Verification items for the finished model (mm, model axes). Face numbers are marked on the shaded views. A direction names the side the tool comes from. Round coordinates to 2 decimals unless told otherwise and drop trailing zeros. Write each loop counter-clockwise with the first axis right and the second up, starting at its lowest first coordinate (ties: lowest second). Pieces come first, ordered by that corner, then holes.
from build123d import *

# Parameters (mm, degrees)
F0_R     = 12.7
F1_DEPTH = 2.032


with BuildPart() as f1:
    # F0 (on Top) → F1 (new body)
    with BuildSketch(Plane.XY):
        Circle(F0_R)
        with BuildLine():
            ThreePointArc((3.175, 0.155574), (4.57905, -1.610295), (5.08, -3.81))
            ThreePointArc((5.08, -3.81), (-2.199705, -8.38905), (-3.175, 0.155574))
            Line((-3.175, 0.155574), (-3.175, 5.08))
            ThreePointArc((-3.175, 5.08), (0, 8.255), (3.175, 5.08))
            Line((3.175, 5.08), (3.175, 0.155574))
        make_face(mode=Mode.SUBTRACT)
    extrude(amount=F1_DEPTH)


solid = f1.part
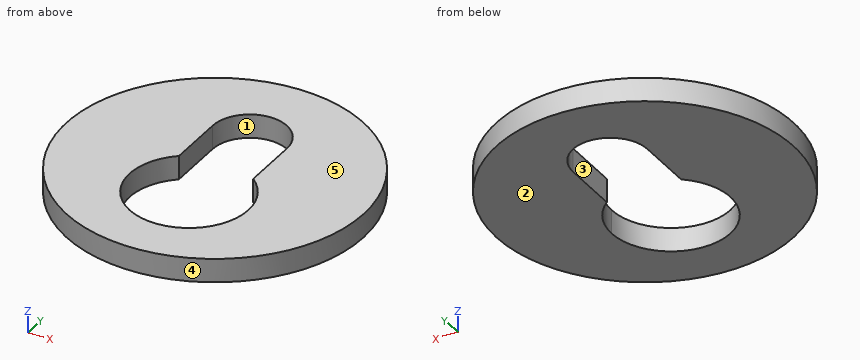
Q1. Release check for a two-part mould opening along Y. For the marked faces 3, 4 and 5 record: released by +Y, released by -Y, zero draft, split by the parting line, or undercut.
Recorded:
face 3: undercut
face 4: split by the parting line
face 5: zero draft
Q2. Sectioned sample at A-A (x = 0). Enter the section's corners in (y, z) (3 decimals).
Recorded:
outline: (-12.7, 0) - (-8.89, 0) - (-8.89, 2.032) - (-12.7, 2.032) - close; (8.255, 0) - (12.7, 0) - (12.7, 2.032) - (8.255, 2.032) - close
Q3. Sectioned sample at B-B (z = 0.5). Enter the section's corners in (x, y) (3 decimals), plus the area to 3 significant figures.
Recorded:
outline: circle Ø25.4 at (0, 0); hole (-3.175, 0.156) arc R5.08 ccw (long way) to (3.175, 0.156) - (3.175, 5.08) arc R3.175 ccw to (-3.175, 5.08) - close
area: 383 mm2
Q4. Sectioned sample at C-C (y = -2.25). Enter the section's corners in (x, z).
Recorded:
outline: (-12.5, 0) - (-4.83, 0) - (-4.83, 2.03) - (-12.5, 2.03) - close; (4.83, 0) - (12.5, 0) - (12.5, 2.03) - (4.83, 2.03) - close
Q5. Sectioned sample at D-D (y = -11). Enter the section's corners in (x, z), plus the area to 3 significant figures.
Recorded:
outline: (-6.35, 0) - (6.35, 0) - (6.35, 2.03) - (-6.35, 2.03) - close
area: 25.8 mm2
Q6. Tool access check on the marked faces 1 and 2. Record the directions out of +Z, -Z, +X, -X, +Y, -Y that give a thin tool (end or side, any length) a straight path to the whole face; none if there is none.
Recorded:
face 1: +Z, -Z
face 2: -Z, +X, -X, +Y, -Y
Q7. Depth check by flat-ended pin: P1, Ø1, axis at x = 7.5, z = 0.5, coming from the +Y side; P2, Ø2, axis at x = -7.5, y = -6, coming from the -Z side; P3, Ø1, axis at y = 3, z = 0.5, coming from the +X side; P4, Ø1, axis at y = 2, z = 1.5, coming from the -X side. Enter the tip coordinate at first touch or a pass-through.
Recorded:
P1: stops at y = 10.6
P2: stops at z = 0
P3: stops at x = 12.45
P4: stops at x = -12.61
Q8. Material ranges on line 1 along Y through (x, z) = (0, 1.15) (3 decimals); line 2 along X through (y, z) = (-3, 1.75) (3 decimals); line 3 along Y through (x, z) = (-2.5, 1.9), recorded low to high.
Recorded:
line 1: y = -12.7 to -8.89, 8.255 to 12.7
line 2: x = -12.341 to -5.015, 5.015 to 12.341
line 3: y = -12.45 to -8.23, 7.04 to 12.45
